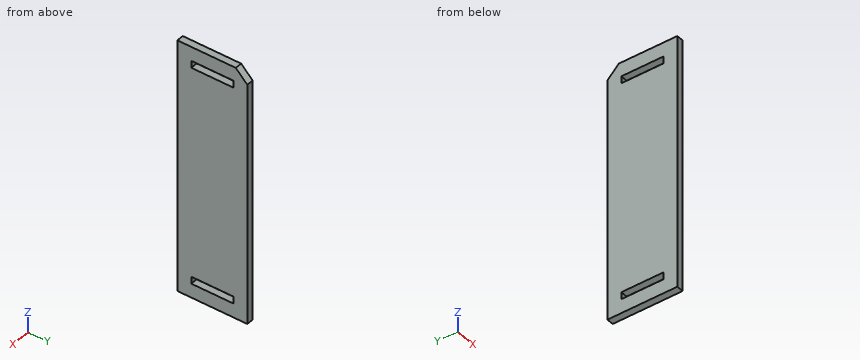
Autodesk Inventor part; units mm, degrees
ref_plane "YZ Plane" through (0, 0, 0) normal (1, 0, 0) x (0, 1, 0)
ref_plane "XZ Plane" through (0, 0, 0) normal (0, 1, 0) x (-1, 0, 0)
ref_plane "XY Plane" through (0, 0, 0) normal (0, 0, 1) x (1, 0, 0)
sketch "Sketch1" plane through (0, 0, 0) normal (1, 0, 0) x (0, 1, 0)
  line L0 (-50, 160) -> (50, 160)
  line L1 (50, 160) -> (50, -160)
  line L2 (50, -160) -> (-50, -160)
  line L3 (-50, -160) -> (-50, 160)
  line L4 (-50, 160) -> (50, -160) construction
  line L5 (50, 160) -> (-50, -160) construction
  point P0 (0, 0)
  dimension "d0" = 320
  dimension "d1" = 100
extrude "Extrusion1" add sketch "Sketch1" along normal blind 10
sketch "Sketch2" plane through (0, 0, 0) normal (-1, 0, 0) x (0, 0, 1)
  line L0 (-160, -50) -> (-160, 50)
  line L1 (160, -50) -> (-160, -50)
  line L2 (160, 50) -> (160, -50)
  line L3 (-160, 50) -> (160, 50)
  line L4 (180, 50) -> (-180, 50)
  line L5 (-180, 50) -> (-180, -50)
  line L6 (-180, -50) -> (180, -50)
  line L7 (180, -50) -> (180, 50)
  line L8 (180, 50) -> (-180, -50) construction
  line L9 (-180, 50) -> (180, -50) construction
  line L10 (150, 30) -> (170, 30)
  line L11 (170, 30) -> (170, -30)
  line L12 (170, -30) -> (150, -30)
  line L13 (150, -30) -> (150, 30)
  line L14 (160, 50) -> (160, -50)
  line L15 (150, 30) -> (170, -30) construction
  line L16 (170, 30) -> (150, -30) construction
  point P0 (0, 0)
  point P1 (160, 0)
  point P2 (160, 30)
  point P3 (160, -30)
  dimension "d4" = 20
  dimension "d5" = 10
  dimension "d6" = 60
extrude "Extrusion2" add sketch "Sketch2" against normal blind 10 contours L2 L12 L11 L10 L4 L7 L6 | L2 L10 L11 L12
extrude "Extrusion3" cut sketch "Sketch2" against normal blind 36.25 contours L12 L13 L10 L2
mirror "Mirror1" about plane through (0, 0, 0) normal (0, 0, 1) of "Extrusion3", "Extrusion2"
chamfer "Chamfer1" distance 16.5 angle 45 1 edges at (5, 50, 180)
properties part number "02_Tam_hong" material "Stainless Steel, Austenitic"
For this review, take the finished solid that the model builds, in its own axes (mm). Give positions to 0.01 mm unless a question says otherwise; leave off trailing zeros. Order: outer loops, then holes, each group sorted by start corner. A loop starts at its lowest first (then second) coordinate and runs counter-clockwise, first axis right, second up.
1) Wall thickness on line 1 (Z direction, x = 5.25, y = 20.5); line 2 (Y direction, x = 6.5, z = 154); line 3 (Z direction, x = 5, y = 34.5): over which ranges is each line inside the solid? List them lowest first.
2) Take a section at B-B (x = 3.5). Give the boundary of the cut face in (y, z), then the cut area to 3 significant figures.
3) Take a section at A-A (y = 0). Give the boundary of the cut face in (x, z).
Derived:
1. line 1: z = -180 to -160, -150 to 150, 160 to 180
1. line 2: y = -50 to -30, 30 to 50
1. line 3: z = -180 to 179
2. outline: (-50, -180) - (50, -180) - (50, 163.5) - (33.5, 180) - (-50, 180) - close; hole (-30, -160) - (30, -160) - (30, -150) - (-30, -150) - close; hole (-30, 150) - (30, 150) - (30, 160) - (-30, 160) - close
2. area: 34,700 mm2
3. outline: (0, -180) - (10, -180) - (10, -160) - (0, -160) - close; (0, -150) - (10, -150) - (10, 150) - (0, 150) - close; (0, 160) - (10, 160) - (10, 180) - (0, 180) - close
